Work out the finished part from the listing and answer in its coordinate system (mm). Face numbers are marked on the shaded views. A direction names the side the tool comes from. Coordinates: 2 decimals unless noted, no trailing zeros. Write each loop counter-clockwise with the first axis right and the second up, starting at its lowest first coordinate (ties: lowest second). Pieces come first, ordered by that corner, then holes. Notation, with made-up numbers: (-19, 5) - (-4, 5) arc R16 ccw to (-4, 29) - close; hole circle Ø3 at (41, 20). An arc over 180 degrees is marked (long way). Use one line per item in the form item = value. Start each with the question number.
Item 1: Determine the mould class of the marked faces 3, 4 and 5 for opening direction X: released by +X, released by -X, zero draft, split by the parting line, or undercut.
Item 2: A cutting plane is placed at A-A (z = 0). Write down the section's boundary in (x, y), then the cut area to 3 significant figures.
Item 3: A cutting plane is placed at B-B (y = 0.85). Write down the section's boundary in (x, z), then the cut area to 3 significant figures.
Item 4: Given pin 1 (1.5 mm diameter, centred on x = -2.5, z = 3, fed in from -Y); pin 2 (1.1 mm diameter, centred on x = -0.5, z = 0, fed in from -Y), each flat-ended and moving along its own axis, determine where each tip first touches the part or whether it passes through.
Item 5: A cutting plane is placed at D-D (x = -2.75). Write down the section's boundary in (y, z), then the cut area to 3 significant figures.
Item 6: Consider probe 1 along X at (y, z) = (2.75, 0); probe 2 along X at (y, z) = (1.7, 0.5). Determine where each line is inside the solid, lowest interval first.
Item 7: A cutting plane is placed at C-C (x = 0). Write down the section's boundary in (y, z).
Item 8: For the marked faces 1 and 2, determine the directions among +Z, -Z, +X, -X, +Y, -Y from which every point of the face is accessible in a straight line to the end or side of a thin tool.
from build123d import *

# Parameters (mm, degrees)
SKETCH_1_R      = 2.9
SKETCH_1_R_2    = 1.9
EXTRUDE_1_DEPTH = 5
EXTRUDE_START   = 5
SKETCH_1_7_R    = 2.9
EXTRUDE_2_DEPTH = 1
SKETCH_1_8_R    = 3.9
SKETCH_1_8_R_2  = 1.9
EXTRUDE_3_DEPTH = 1


with BuildPart() as part:
    # 草图1 → 凸台-拉伸1 (new body)
    with BuildSketch(Plane(origin=(0, 0, 0), x_dir=(1, 0, 0), z_dir=(0, 1, 0))):
        with Locations(Location((0, 0, 0), (0, 0, 270))):
            Circle(SKETCH_1_R)
        with Locations(Location((0, 0, 0), (0, 0, 270))):
            Circle(SKETCH_1_R_2, mode=Mode.SUBTRACT)
    extrude(amount=EXTRUDE_1_DEPTH)

    # 草图1<7> → 凸台-拉伸2 (add)
    with BuildSketch(Plane(origin=(0, 0, 0), x_dir=(1, 0, 0), z_dir=(0, 1, 0)).offset(EXTRUDE_START)):
        with Locations(Location((0, 0, 0), (0, 0, 270))):
            Circle(SKETCH_1_7_R)
    extrude(amount=EXTRUDE_2_DEPTH)

    # 草图1<8> → 凸台-拉伸3 (add)
    with BuildSketch(Plane(origin=(0, 0, 0), x_dir=(1, 0, 0), z_dir=(0, 1, 0))):
        with Locations(Location((0, 0, 0), (0, 0, 270))):
            Circle(SKETCH_1_8_R)
        with Locations(Location((0, 0, 0), (0, 0, 270))):
            Circle(SKETCH_1_8_R_2, mode=Mode.SUBTRACT)
    extrude(amount=EXTRUDE_3_DEPTH)


solid = part.part
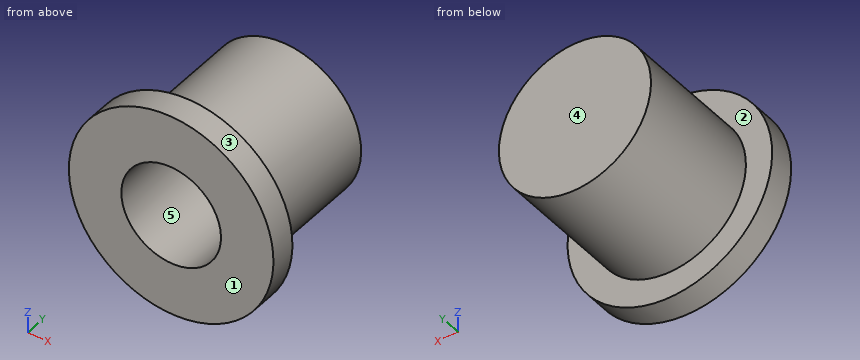
Answer:
q1.face_3 = split by the parting line
q1.face_4 = zero draft
q1.face_5 = undercut
q2.outline = (-3.9, 0) - (-1.9, 0) - (-1.9, 5) - (1.9, 5) - (1.9, 0) - (3.9, 0) - (3.9, 1) - (2.9, 1) - (2.9, 6) - (-2.9, 6) - (-2.9, 1) - (-3.9, 1) - close
q2.area = 17.8 mm²
q3.outline = circle Ø7.8 at (0, 0); hole circle Ø3.8 at (0, 0)
q3.area = 36.4 mm²
q4.pin_1 = 0
q4.pin_2 = 5
q5.outline = (0, -2.77) - (1, -2.77) - (1, -0.92) - (6, -0.92) - (6, 0.92) - (1, 0.92) - (1, 2.77) - (0, 2.77) - close
q5.area = 14.7 mm²
q6.probe_1 = -2.9 to -1.9, 1.9 to 2.9
q6.probe_2 = -2.86 to -1.83, 1.83 to 2.86
q7.outline = (0, -3.9) - (1, -3.9) - (1, -2.9) - (6, -2.9) - (6, 2.9) - (1, 2.9) - (1, 3.9) - (0, 3.9) - (0, 1.9) - (5, 1.9) - (5, -1.9) - (0, -1.9) - close
q8.face_1 = +Z, -Z, +X, -X, -Y
q8.face_2 = +Y
